Read the model definition and answer for the solid it produces. Units are mm, in the model's axes. A direction names the side the tool comes from. Give positions to 0.01 mm unless a question says otherwise; leave off trailing zeros. Order: outer loops, then holes, each group sorted by start corner. A loop starts at its lowest first (then second) coordinate and runs counter-clockwise, first axis right, second up. Notation, with made-up numbers: (63.5, 5.5) - (108.5, 5.5) arc R13 cw to (108.5, 20.5) - close; hole circle Ø2 at (-8.75, -8). An arc over 180 degrees is marked (long way). Write item = value, one per line.
```python
from build123d import *

# Parameters (mm, degrees)
F0_W     = 400
F0_H     = 400
F0_W_2   = 350
F0_H_2   = 350
F1_DEPTH = 3
F2_W     = 400
F2_H     = 400
F2_W_2   = 394
F2_H_2   = 394
F3_DEPTH = 70
F4_W     = 20
F4_H     = 20
F5_DEPTH = 30
F6_W     = 50
F6_H     = 50
F7_DEPTH = 3


with BuildPart() as f1:
    # F0 (on Top) → F1 (new body)
    with BuildSketch(Plane.XY):
        Rectangle(F0_W, F0_H)
        Rectangle(F0_W_2, F0_H_2, mode=Mode.SUBTRACT)
    extrude(amount=F1_DEPTH)

    # F2 (on face) → F3 (join)
    with BuildSketch(Plane.XY.offset(3)):
        Rectangle(F2_W, F2_H)
        Rectangle(F2_W_2, F2_H_2, mode=Mode.SUBTRACT)
    extrude(amount=F3_DEPTH)

    # F4 (on face) → F5 (join)
    with BuildSketch(Plane(origin=(0, 0, 0), x_dir=(1, 0, 0), z_dir=(0, 0, -1))):
        with Locations((-190, 190)):
            Rectangle(F4_W, F4_H)
        with Locations((190, 190)):
            Rectangle(F4_W, F4_H)
        with Locations((-190, -190)):
            Rectangle(F4_W, F4_H)
        with Locations((190, -190)):
            Rectangle(F4_W, F4_H)
    extrude(amount=F5_DEPTH)

    # F6 (on face) → F7 (join)
    with BuildSketch(Plane(origin=(0, 0, -30), x_dir=(1, 0, 0), z_dir=(0, 0, -1))):
        with Locations((-190, 190)):
            Rectangle(F6_W, F6_H)
        with Locations((190, 190)):
            Rectangle(F6_W, F6_H)
        with Locations((190, -190)):
            Rectangle(F6_W, F6_H)
        with Locations((-190, -190)):
            Rectangle(F6_W, F6_H)
    extrude(amount=F7_DEPTH)


solid = f1.part
```
1. Section A-A (z = 21) is taken. Determine the outline of the cut face in (x, y).
Recorded:
outline = (-200, -200) - (200, -200) - (200, 200) - (-200, 200) - close; hole (-197, -197) - (197, -197) - (197, 197) - (-197, 197) - close
2. For faces 1 (the face through (-3, 197, 38)), 2 (the face through (200, -3, 32)), 3 (the face through (190, -180, -15)), determine the directions among +Z, -Z, +X, -X, +Y, -Y from which every point of the face is accessible in a straight line to the end or side of a thin tool.
Recorded:
face_1 = +Z
face_2 = +Z, +X, +Y, -Y
face_3 = +X, -X
3. Straight lines are drawn through the part: L1, parallel to X at y = -141, z = 22; L2, parallel to X at y = 193, z = -10.5. For each, find the intervals that lie inside material, in ascending order. Write a range as [from, to].
Recorded:
L1 = [-200, -197], [197, 200]
L2 = [-200, -180], [180, 200]
4. Section D-D (z = -12.5) is taken. Determine the outline of the cut face in (x, y), and give its area (3 significant figures).
Recorded:
outline = (-200, -200) - (-180, -200) - (-180, -180) - (-200, -180) - close; (-200, 180) - (-180, 180) - (-180, 200) - (-200, 200) - close; (180, -200) - (200, -200) - (200, -180) - (180, -180) - close; (180, 180) - (200, 180) - (200, 200) - (180, 200) - close
area = 1,600 mm^2
5. Section B-B (y = -133) is taken. Determine the outline of the cut face in (x, z), and give its area (3 significant figures).
Recorded:
outline = (-200, 0) - (-175, 0) - (-175, 3) - (-197, 3) - (-197, 73) - (-200, 73) - close; (175, 0) - (200, 0) - (200, 73) - (197, 73) - (197, 3) - (175, 3) - close
area = 570 mm^2
6. Determine the mould class of faces 4 (the face through (180, 190, -15)), 5 (the face through (-190, -190, -33)), 6 (the face through (197, -3, 38)) for opening direction Z: +Z half, -Z half, draft (parallel to the pull), parting line (faces both ways), or undercut.
Recorded:
face_4 = undercut
face_5 = -Z half
face_6 = draft
7. Flat-ended cylindrical pins translate along their axes: pin 1 (6 mm diameter, centred on y = 30.5, z = 52.5, fed in from +X); pin 2 (4 mm diameter, centred on x = 70.5, z = 16.5, fed in from +Y); pin 3 (22 mm diameter, centred on x = 194, z = -13.5, fed in from -Y). Find the tip coordinate at first contact, or state that the pin passes through.
Recorded:
pin_1 = 200
pin_2 = 200
pin_3 = -200
